Drawing for the job (mm, zero at the part's lowest x, y, z). Give positions to 0.01 mm unless a question says otherwise; leave off trailing zeros. Loops run counter-clockwise (first coordinate to the right, second up) from the corner with the lowest first, then second, coordinate; pieces in that order, holes last. Notation, with made-up numbers: M -35,-27 L 19,-27 A28 cw 19,-1 Z; hole C 80.25,72 d7. An arc over 180 degrees is marked long. Answer in a Markdown table with one row per item. Add a question column.
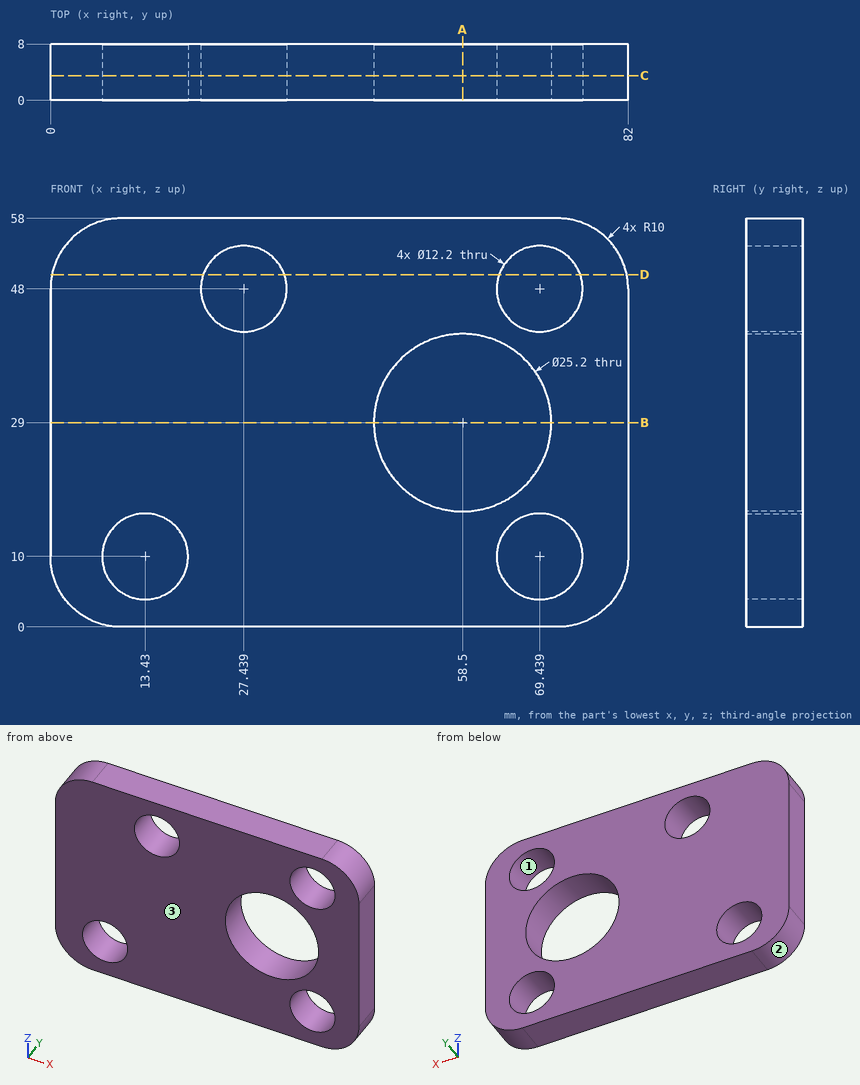
(1) Pull direction Z, two halves, no side cores. Call the marked faces 1, 2 and 3: +Z half, -Z half, draft (parallel to the pull), parting line (faces both ways), or undercut.
(2) Pin check, flat tip, straight feed: pin 1 (14 mm diameter, centred on x = 13.43, z = 10, fed in from +Y). Stop position of the tip, or through.
(3) Slice it at B-B, the plane z = 29. Give the cut face in (x, y).
(4) Slice it at D-D, the plane z = 50. Give the cut face in (x, y), then the cut area to 3 significant figures.
(5) Slice it at A-A, the plane x = 58.5. Give the cut face in (y, z), then the cut area to 3 significant figures.
(6) Slice it at C-C, the plane y = 3.5. Give the cut face in (x, z).
(7) Wall check: line 1 (X direction, y = 2.25, z = 48); line 2 (X direction, y = 4.75, z = 10.5); line 3 (X direction, y = 4, z = 29). Give the ranges that are in metal, low to high.
Solution:
| question | item | result |
|---|---|---|
| 1 | face 1 | undercut |
| 1 | face 2 | -Z half |
| 1 | face 3 | draft |
| 2 | pin 1 | y = 8 |
| 3 | outline | M 0,0 L 45.9,0 L 45.9,8 L 0,8 Z; M 71.1,0 L 82,0 L 82,8 L 71.1,8 Z |
| 4 | outline | M 0.2,0 L 21.68,0 L 21.68,8 L 0.2,8 Z; M 33.2,0 L 63.68,0 L 63.68,8 L 33.2,8 Z; M 75.2,0 L 81.8,0 L 81.8,8 L 75.2,8 Z |
| 4 | area | 468 mm^2 |
| 5 | outline | M 0,0 L 8,0 L 8,16.4 L 0,16.4 Z; M 0,41.6 L 8,41.6 L 8,58 L 0,58 Z |
| 5 | area | 262 mm^2 |
| 6 | outline | M 0,10 A10 ccw 10,0 L 72,0 A10 ccw 82,10 L 82,48 A10 ccw 72,58 L 10,58 A10 ccw 0,48 Z; hole C 13.43,10 d12.2; hole C 27.44,48 d12.2; hole C 58.5,29 d25.2; hole C 69.44,10 d12.2; hole C 69.44,48 d12.2 |
| 7 | line 1 | 0 to 21.34, 33.54 to 63.34, 75.54 to 82 |
| 7 | line 2 | 0 to 7.35, 19.51 to 63.36, 75.52 to 82 |
| 7 | line 3 | 0 to 45.9, 71.1 to 82 |
